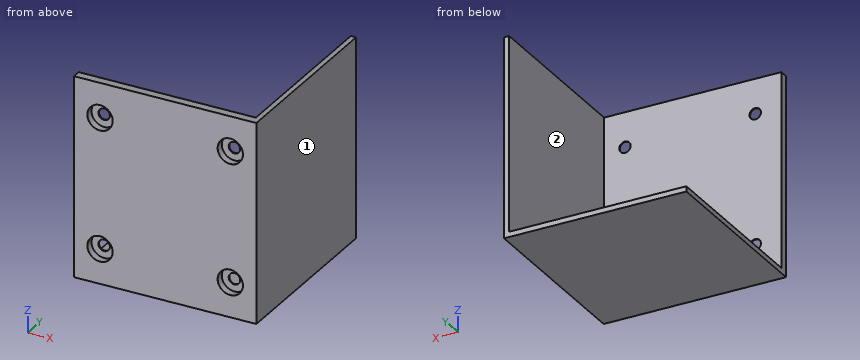
```python
from build123d import *

# Parameters (mm, degrees)
SKETCH3_W                              = 105
SKETCH3_H                              = 115
BOSS_EXTRUDE1_DEPTH                    = 105
SKETCH6_W                              = 102
SKETCH6_H                              = 112
CUT_EXTRUDE1_DEPTH                     = 100
CBORE_FOR_M6_HEX_HEAD_BOLT1_AT_2_COUNT = 2
CBORE_FOR_M6_HEX_HEAD_BOLT1_AT_2_PITCH = 75
CBORE_FOR_M6_HEX_HEAD_BOLT1_AT_3_COUNT = 2
CBORE_FOR_M6_HEX_HEAD_BOLT1_AT_3_PITCH = 106.066017178
CBORE_FOR_M6_HEX_HEAD_BOLT1_AT_4_COUNT = 2
CBORE_FOR_M6_HEX_HEAD_BOLT1_AT_4_PITCH = 75


with BuildPart() as part:
    # Sketch3 → Boss-Extrude1 (new body)
    with BuildSketch(Plane(origin=(0, 0, 0), x_dir=(1, 0, 0), z_dir=(0, 1, 0))):
        Rectangle(SKETCH3_W, SKETCH3_H)
    extrude(amount=BOSS_EXTRUDE1_DEPTH)

    # Sketch6 → Cut-Extrude1 (cut)
    with BuildSketch(Plane(origin=(0, 105, 0), x_dir=(1, 0, 0), z_dir=(0, 1, 0))):
        with Locations((-1.5, -1.5)):
            Rectangle(SKETCH6_W, SKETCH6_H)
    extrude(amount=-CUT_EXTRUDE1_DEPTH, mode=Mode.SUBTRACT)

    # Sketch7 → CBORE for M6 Hex Head Bolt1 (revolve, cut)
    with BuildSketch(Plane(origin=(37.5, 0, 37.5), x_dir=(0, 0, -1), z_dir=(1, 0, 0))):
        Polygon((0, 0), (0, 105), (3.3, 105), (3.3, 4.38), (7.275, 4.38), (7.275, 0.025), (7.3, 0), align=None)
    cbore_for_m6_hex_head_bolt1 = revolve(axis=Axis((37.5, -6.35, 37.5), (0, 1, 0)), mode=Mode.SUBTRACT)

    # CBORE for M6 Hex Head Bolt1 at 2: CBORE for M6 Hex Head Bolt1 ×2
    with Locations(*[(0, 0, -i * CBORE_FOR_M6_HEX_HEAD_BOLT1_AT_2_PITCH) for i in range(1, CBORE_FOR_M6_HEX_HEAD_BOLT1_AT_2_COUNT)]):
        add(cbore_for_m6_hex_head_bolt1, mode=Mode.SUBTRACT)

    # CBORE for M6 Hex Head Bolt1 at 3: CBORE for M6 Hex Head Bolt1 ×2
    with Locations(*[Vector(-0.7071067811865476, 0, -0.7071067811865476) * (i * CBORE_FOR_M6_HEX_HEAD_BOLT1_AT_3_PITCH) for i in range(1, CBORE_FOR_M6_HEX_HEAD_BOLT1_AT_3_COUNT)]):
        add(cbore_for_m6_hex_head_bolt1, mode=Mode.SUBTRACT)

    # CBORE for M6 Hex Head Bolt1 at 4: CBORE for M6 Hex Head Bolt1 ×2
    with Locations(*[(-i * CBORE_FOR_M6_HEX_HEAD_BOLT1_AT_4_PITCH, 0, 0) for i in range(1, CBORE_FOR_M6_HEX_HEAD_BOLT1_AT_4_COUNT)]):
        add(cbore_for_m6_hex_head_bolt1, mode=Mode.SUBTRACT)


solid = part.part
```
Geometry check sheet. Reference: the model listing, model coordinates, mm. Face numbers are marked on the shaded views. A direction names the side the tool comes from. Round coordinates to 2 decimals unless told otherwise and drop trailing zeros. Loops run counter-clockwise (first coordinate to the right, second up) from the corner with the lowest first, then second, coordinate; pieces in that order, holes last. Notation, with made-up numbers: M 49,35.5 L 62,35.5 A23 cw 62,62.5 Z; hole C 70.25,-22 d11. An arc over 180 degrees is marked long. Return JSON: item names as keys, results as strings. Group by question number.
(1) Section check B-B, the plane z = -37.5. Enter the section's corners in (x, y) (3 decimals), and give its area (3 significant figures).
(2) Set-up check for the marked faces 1 and 2: record each of +Z, -Z, +X, -X, +Y, -Y from which the full face is reachable in a straight line by a thin tool's end or side.
(3) Scan lines: line 1 along Z through (x, y) = (-37.5, 1.85) (3 decimals); line 2 along X through (y, z) = (4.55, -37.5); line 3 along X through (y, z) = (4, 37). Record each from-to range of solid material in increasing order. Write a range as [from, to].
(4) Section check A-A, the plane x = 37.5. Enter the section's corners in (y, z) (3 decimals), and give its area (3 significant figures).
(5) Section check D-D, the plane y = 80. Enter the section's corners in (x, z).
(6) Section check C-C, the plane x = -10. Enter the section's corners in (y, z).
(7) Go/stop test with flat-tipped pins: pin 1 (10 mm diameter, centred on x = 20, y = 40, fed in from +Z); pin 2 (23.5 mm diameter, centred on x = -37.5, z = -37.5, fed in from +Y); pin 3 (8 mm diameter, centred on y = 22, z = 11, fed in from -X). Record where each tip stops, or that it passes through.
Data:
{
 "1": {"outline": "M -52.5,0 L -44.8,0 L -44.775,0.025 L -44.775,4.38 L -40.8,4.38 L -40.8,5 L -52.5,5 Z; M -34.2,4.38 L -30.225,4.38 L -30.225,0.025 L -30.2,0 L 30.2,0 L 30.225,0.025 L 30.225,4.38 L 34.2,4.38 L 34.2,5 L -34.2,5 Z; M 40.8,4.38 L 44.775,4.38 L 44.775,0.025 L 44.8,0 L 52.5,0 L 52.5,105 L 49.5,105 L 49.5,5 L 40.8,5 Z", "area": "689 mm²"},
 "2": {"face 1": "+Z, -Z, +X, +Y, -Y", "face 2": "+Z, -X, +Y"},
 "3": {"line 1": "[-57.5, -44.775], [-30.225, 30.225], [44.775, 57.5]", "line 2": "[-52.5, -40.8], [-34.2, 34.2], [40.8, 52.5]", "line 3": "[-52.5, -44.76], [-30.24, 30.24], [44.76, 52.5]"},
 "4": {"outline": "M 0,-57.5 L 105,-57.5 L 105,-54.5 L 5,-54.5 L 5,-40.8 L 4.38,-40.8 L 4.38,-44.775 L 0.025,-44.775 L 0,-44.8 Z; M 0,-30.2 L 0.025,-30.225 L 4.38,-30.225 L 4.38,-34.2 L 5,-34.2 L 5,34.2 L 4.38,34.2 L 4.38,30.225 L 0.025,30.225 L 0,30.2 Z; M 0,44.8 L 0.025,44.775 L 4.38,44.775 L 4.38,40.8 L 5,40.8 L 5,57.5 L 0,57.5 Z", "area": "739 mm²"},
 "5": {"outline": "M -52.5,-57.5 L 52.5,-57.5 L 52.5,57.5 L 49.5,57.5 L 49.5,-54.5 L -52.5,-54.5 Z"},
 "6": {"outline": "M 0,-57.5 L 105,-57.5 L 105,-54.5 L 5,-54.5 L 5,57.5 L 0,57.5 Z"},
 "7": {"pin 1": "z = -54.5", "pin 2": "y = 5", "pin 3": "x = 49.5"}
}
